Geometry check sheet. Reference: the model listing, model coordinates, mm. A direction names the side the tool comes from. Coordinates: 2 decimals unless noted, no trailing zeros. Write each loop counter-clockwise with the first axis right and the second up, starting at its lowest first coordinate (ties: lowest second). Pieces come first, ordered by that corner, then holes.
from build123d import *

# Parameters (mm, degrees)
SKETCH1_W           = 50
SKETCH1_H           = 55
BOSS_EXTRUDE1_DEPTH = 68
SKETCH3_R           = 21.125
CUT_EXTRUDE1_DEPTH  = 50
SKETCH2_R           = 14
SKETCH2_R_2         = 2
CUT_EXTRUDE2_DEPTH  = 91.96153033
SKETCH4_W           = 19.1
SKETCH4_H           = 17.5
CUT_EXTRUDE3_DEPTH  = 89.770772217
SKETCH5_R           = 2
CUT_EXTRUDE4_DEPTH  = 91.96153033


with BuildPart() as part:
    # Sketch1 → Boss-Extrude1 (new body)
    with BuildSketch(Plane(origin=(0, 0, 0), x_dir=(1, 0, 0), z_dir=(0, 1, 0))):
        Rectangle(SKETCH1_W, SKETCH1_H)
    extrude(amount=BOSS_EXTRUDE1_DEPTH)

    # Sketch3 → Cut-Extrude1 (cut)
    with BuildSketch(Plane(origin=(0, 0, -27.5), x_dir=(-1, 0, 0), z_dir=(0, 0, -1))):
        with Locations((0, 42.5)):
            Circle(SKETCH3_R)
    extrude(amount=-CUT_EXTRUDE1_DEPTH, mode=Mode.SUBTRACT)

    # Sketch2 → Cut-Extrude2 (cut, through all)
    with BuildSketch(Plane.XY.offset(27.5)):
        with Locations((0, 42.5)):
            Circle(SKETCH2_R)
        with Locations((0, 60)):
            Circle(SKETCH2_R_2)
        with Locations((17.5, 42.5)):
            Circle(SKETCH2_R_2)
        with Locations((0, 25)):
            Circle(SKETCH2_R_2)
        with Locations((-17.5, 42.5)):
            Circle(SKETCH2_R_2)
    extrude(amount=-CUT_EXTRUDE2_DEPTH, mode=Mode.SUBTRACT)

    # Sketch4 → Cut-Extrude3 (cut, through all)
    with BuildSketch(Plane(origin=(25, 0, 0), x_dir=(0, 0, -1), z_dir=(1, 0, 0))):
        with Locations((0, 8.75)):
            Rectangle(SKETCH4_W, SKETCH4_H)
    extrude(amount=-CUT_EXTRUDE3_DEPTH, mode=Mode.SUBTRACT)

    # Sketch5 → Cut-Extrude4 (cut, through all)
    with BuildSketch(Plane.XY.offset(27.5)):
        with Locations((-16.8, 8)):
            Circle(SKETCH5_R)
        with Locations((-5.6, 8)):
            Circle(SKETCH5_R)
        with Locations((5.6, 8)):
            Circle(SKETCH5_R)
        with Locations((16.8, 8)):
            Circle(SKETCH5_R)
    extrude(amount=-CUT_EXTRUDE4_DEPTH, mode=Mode.SUBTRACT)


solid = part.part
1. Thickness scan on line 1 along Y through (x, z) = (0, 23.95); line 2 along X through (y, z) = (43, 3.5); line 3 along Z through (x, y) = (-18, 13.5). Record the ranges inside material, lowest first.
Computed values:
line 1: y = 0 to 23, 27 to 28.5, 56.5 to 58, 62 to 68
line 2: x = -25 to -21.12, 21.12 to 25
line 3: z = -27.5 to -9.55, 9.55 to 27.5
2. Gauge pin test, flat ends, axial feed: pin 1 Ø9.5 at (x, z) = (-4.5, 1) entering from -Y; pin 2 Ø6 at (x, y) = (12, 32) entering from -Z. Record the tip position at first contact, or that the pin passes through.
Computed values:
pin 1: stops at y = 17.5
pin 2: stops at z = 22.5
3. Sectioned sample at A-A, the plane y = 14. Record the boundary of the cut face in (x, z).
Computed values:
outline: (-25, -27.5) - (25, -27.5) - (25, -9.55) - (-25, -9.55) - close; (-25, 9.55) - (25, 9.55) - (25, 27.5) - (-25, 27.5) - close
4. Sectioned sample at B-B, the plane x = 0. Record the boundary of the cut face in (y, z) (3 decimals).
Computed values:
outline: (0, -27.5) - (21.375, -27.5) - (21.375, 22.5) - (23, 22.5) - (23, 27.5) - (0, 27.5) - (0, 9.55) - (17.5, 9.55) - (17.5, -9.55) - (0, -9.55) - close; (27, 22.5) - (28.5, 22.5) - (28.5, 27.5) - (27, 27.5) - close; (56.5, 22.5) - (58, 22.5) - (58, 27.5) - (56.5, 27.5) - close; (62, 22.5) - (63.625, 22.5) - (63.625, -27.5) - (68, -27.5) - (68, 27.5) - (62, 27.5) - close
5. Draft check along X on faces 1 (the flat face through (0, 18, -27.5)), 2 (the cylindrical face through (17.066, 40.548, 25.035)), 3 (the flat face through (-25, 34, 0)). Enter one of: released by +X, released by -X, zero draft, split by the parting line, or undercut.
Computed values:
face 1: zero draft
face 2: undercut
face 3: released by -X
6. Access from +Z, -Z, +X, -X, +Y, -Y to the whole of each face (thin tool, end or side, straight path). Record for faces 4 (the flat face through (-4.4, 28.7, 22.5)), 5 (the flat face through (-6, 26, 27.5)), 6 (the flat face through (0, 9, 9.55)).
Computed values:
face 4: -Z
face 5: +Z, +X, -X, +Y, -Y
face 6: +X, -X, -Y
7. Sectioned sample at D-D, the plane z = -8. Record the boundary of the cut face in (x, y) (3 decimals), and give its area (3 significant figures).
Computed values:
outline: (-25, 17.5) - (25, 17.5) - (25, 68) - (-25, 68) - close; hole circle Ø42.25 at (0, 42.5)
area: 1,120 mm2
8. Sectioned sample at C-C, the plane z = 17.5. Record the boundary of the cut face in (x, y) (3 decimals).
Computed values:
outline: (-25, 0) - (25, 0) - (25, 68) - (-25, 68) - close; hole circle Ø42.25 at (0, 42.5); hole circle Ø4 at (-16.8, 8); hole circle Ø4 at (-5.6, 8); hole circle Ø4 at (5.6, 8); hole circle Ø4 at (16.8, 8)
